```python
from build123d import *

# Parameters (mm, degrees)
SKETCH1_R           = 5.53085
SKETCH1_W           = 11.811
SKETCH1_H           = 3.175
BOSS_EXTRUDE1_DEPTH = 2.54
SKETCH1_3_W         = 16.150142566
SKETCH1_3_H         = 6.574737844
BOSS_EXTRUDE2_DEPTH = 10.16
BOSS_EXTRUDE3_START = -5.08
BOSS_EXTRUDE3_DEPTH = 5.08
BOSS_EXTRUDE5_DEPTH = 2.032


with BuildPart() as part:
    # Sketch1 → Boss-Extrude1 (new body)
    with BuildSketch(Plane(origin=(0, 0, 0), x_dir=(1, 0, 0), z_dir=(0, 1, 0))):
        with BuildLine():
            ThreePointArc((13.753578899, 4.597841674), (0, 5.078127233), (-13.753578899, 4.597841674))
            Line((-13.753578899, 4.597841674), (-13.39934665, -0.467915496))
            Line((-13.39934665, -0.467915496), (-13.39934665, -22.557024998))
            Line((-13.39934665, -22.557024998), (13.39934665, -22.557024998))
            Line((13.39934665, -22.557024998), (13.39934665, -0.467915496))
            Line((13.39934665, -0.467915496), (13.753578899, 4.597841674))
        make_face()
        with Locations(Location((0, -13.62075, 0), (0, 0, 270))):
            Circle(SKETCH1_R, mode=Mode.SUBTRACT)
        with Locations((0, -3.5433)):
            Rectangle(SKETCH1_W, SKETCH1_H, mode=Mode.SUBTRACT)
    extrude(amount=BOSS_EXTRUDE1_DEPTH)

    # Sketch1_3 → Boss-Extrude2 (add)
    with BuildSketch(Plane(origin=(0, 0, 0), x_dir=(1, 0, 0), z_dir=(0, 1, 0))):
        with Locations((0, -3.6068)):
            Rectangle(SKETCH1_3_W, SKETCH1_3_H)
        Polygon((0, -5.1308), (-5.9055, -5.1308), (-5.9055, -1.9558), (5.9055, -1.9558), (5.9055, -5.1308), align=None, mode=Mode.SUBTRACT)
    extrude(amount=BOSS_EXTRUDE2_DEPTH)

    # Sketch1_4 → Boss-Extrude3 (add)
    with BuildSketch(Plane(origin=(0, 0, 0), x_dir=(1, 0, 0), z_dir=(0, 1, 0)).offset(BOSS_EXTRUDE3_START)):
        with BuildLine():
            ThreePointArc((-13.753578899, 4.597841674), (0, 5.078127233), (13.753578899, 4.597841674))
            Line((13.753578899, 4.597841674), (13.39934665, -0.467915496))
            ThreePointArc((13.39934665, -0.467915496), (6.703757073, -0.117014515), (0, 0))
            ThreePointArc((0, 0), (-6.703757073, -0.117014515), (-13.39934665, -0.467915496))
            Line((-13.39934665, -0.467915496), (-13.753578899, 4.597841674))
        make_face()
    extrude(amount=BOSS_EXTRUDE3_DEPTH)

    # Sketch2 → Boss-Extrude5 (add)
    with BuildSketch(Plane.XZ.offset(5.08)):
        Polygon((-13.753578899, -4.597841674), (-13.39934665, 0.467915496), (-13.300671129, 1.879041191), (13.300671129, 1.879041191), (13.39934665, 0.467915496), (13.753578899, -4.597841674), align=None)
    extrude(amount=-BOSS_EXTRUDE5_DEPTH)


solid = part.part
```
Input: part model. Units: mm. Frame: model coordinates. A direction names the side the tool comes from. Coordinates: 2 decimals unless noted, no trailing zeros. Loops run counter-clockwise (first coordinate to the right, second up) from the corner with the lowest first, then second, coordinate; pieces in that order, holes last. Notation, with made-up numbers: (15.25, 55.5) - (43.25, 55.5) arc R6 cw to (43.25, 60.5) - close; hole circle Ø7 at (12.5, 63.5). An arc over 180 degrees is marked (long way). Answer in a Markdown table with one row per item.
(1) Cut plane C-C on x = -8.5. Output: boundary loops of the cut face in (y, z), plus the area to 3 significant figures.
Model answer:
| item | result |
|---|---|
| outline | (-5.08, -4.89) - (2.54, -4.89) - (2.54, 22.56) - (0, 22.56) - (0, 0.19) - (-3.05, 0.19) - (-3.05, 1.88) - (-5.08, 1.88) - close |
| area | 99.0 mm² |
(2) Cut plane D-D on z = 17.5. Output: boundary loops of the cut face in (x, y).
Model answer:
| item | result |
|---|---|
| outline | (-13.4, 0) - (-3.94, 0) - (-3.94, 2.54) - (-13.4, 2.54) - close; (3.94, 0) - (13.4, 0) - (13.4, 2.54) - (3.94, 2.54) - close |
(3) Mould query, pull axis X, two halves, no side actions, for faces 4 (the face through (0, 5, 5.131)), 5 (the face through (-0.19, -1.32, -5.08)), 6 (the face through (0, 6, 0.319)). Classes: pulls with the +X half, pulls with the -X half, needs draft (parallel to the pull), parting line crosses it, or undercut.
Model answer:
| item | result |
|---|---|
| face 4 | undercut |
| face 5 | parting line crosses it |
| face 6 | needs draft |
(4) Pin query (flat end, axial travel): P1, Ø10, axis at x = 9, z = 10.5, coming from the +Y side; P2, Ø1, axis at x = -5.5, y = -4, coming from the +Z side; P3, Ø1, axis at x = 10, z = 9, coming from the -Y side; P4, Ø8, axis at x = 0, y = 5, coming from the -Z side. Return the tip coordinate at first contact, or that it passes through.
Model answer:
| item | result |
|---|---|
| P1 | stops at y = 10.16 |
| P2 | stops at z = 1.88 |
| P3 | stops at y = 0 |
| P4 | stops at z = -5.08 |
(5) Cut plane A-A on z = 4.25. Output: boundary loops of the cut face in (x, y), plus the area to 3 significant figures.
Model answer:
| item | result |
|---|---|
| outline | (-13.4, 0) - (-5.91, 0) - (-5.91, 10.16) - (-8.08, 10.16) - (-8.08, 2.54) - (-13.4, 2.54) - close; (5.91, 0) - (13.4, 0) - (13.4, 2.54) - (8.08, 2.54) - (8.08, 10.16) - (5.91, 10.16) - close |
| area | 71.1 mm² |
(6) Material intervals for L1, parallel to Z at x = 0.5, y = 3.5; L2, parallel to Z at x = -2.5, y = 2.25; L3, parallel to X at y = 7.5, z = 1.5, sorted ascending. Write a range as from..to.
Model answer:
| item | result |
|---|---|
| L1 | z = 0.32..1.96, 5.13..6.89 |
| L2 | z = -5.06..1.96, 5.13..8.69, 18.55..22.56 |
| L3 | x = -8.08..8.08 |
(7) Set-up query: faces 1 (the face through (0, -4, 1.879)), 2 (the face through (0, -3.048, 1)), 3 (the face through (-5.906, 5, 4)). Return all of +Z, -Z, +X, -X, +Y, -Y with unobstructed straight access to the full face (end or side cutting, diameter ignored); none if empty.
Model answer:
| item | result |
|---|---|
| face 1 | +Z, +X, -X, -Y |
| face 2 | +Z |
| face 3 | +Y, -Y |
(8) Cut plane B-B on y = 5.25. Output: boundary loops of the cut face in (x, z), plus the area to 3 significant figures.
Model answer:
| item | result |
|---|---|
| outline | (-8.08, 0.32) - (8.08, 0.32) - (8.08, 6.89) - (-8.08, 6.89) - close; hole (-5.91, 1.96) - (5.91, 1.96) - (5.91, 5.13) - (-5.91, 5.13) - close |
| area | 68.7 mm² |
